Input: dimensioned drawing with shaded views. Units: mm. Origin: part minimum x, y, z. A direction names the side the tool comes from. Give positions to 0.01 mm unless a question says otherwise; leave off trailing zeros. Order: outer loops, then holes, each group sorted by start corner. A loop starts at its lowest first (then second) coordinate and runs counter-clockwise, first axis right, second up. Notation, with made-up numbers: (-38.5, -22.75) -> (4.5, -22.75) arc R26 ccw to (4.5, -5.75) -> close; hole circle Ø5 at (25.25, 17.5). An arc over 180 degrees is marked (long way). One line per question, with ' | ' between items. Start each with the question number.
(1) Set-up query: the marked faces 1, 2 and 3. Return all of +Z, -Z, +X, -X, +Y, -Y with unobstructed straight access to the full face (end or side cutting, diameter ignored); none if empty.
(2) Ray query, L1, parallel to Y at x = 19.5, z = 4.7. Return the intervals inside material, ascending.
(3) First-contact query: pin 1 Ø2.5 at (y, z) = (62, 3.5) entering from +X; pin 2 Ø1.5 at (x, z) = (45.5, 2) entering from +Y. Flat tips, straight axial feed; report the tip coordinate or a pass-through.
(4) Section A-A (z = 2.3). Return loops of the section in (x, y).
(5) Section B-B (x = 40.5). Return loops of the section in (y, z).
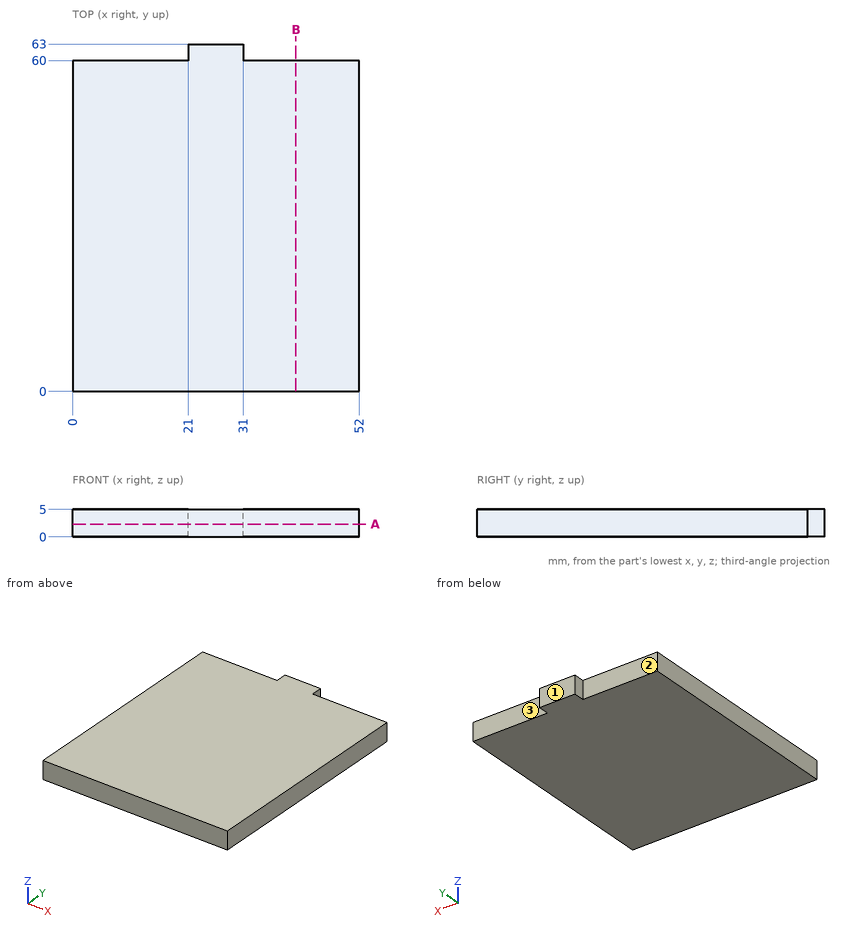
Response:
1) face 1: +Z, -Z, +X, -X, +Y | face 2: +Z, -Z, -X, +Y | face 3: +Z, -Z, +X, +Y
2) L1: y = 0 to 60
3) pin 1: stops at x = 31 | pin 2: stops at y = 60
4) outline: (0, 0) -> (52, 0) -> (52, 60) -> (31, 60) -> (31, 63) -> (21, 63) -> (21, 60) -> (0, 60) -> close
5) outline: (0, 0) -> (60, 0) -> (60, 5) -> (0, 5) -> close
